Could you check a few things on this model? Use its own coordinates, in mm. Face numbers are marked on the shaded views. A direction names the side the tool comes from. Give positions to 0.01 mm unless a question says otherwise; leave off trailing zeros. Write each loop counter-clockwise with the first axis right and the second up, starting at its lowest first coordinate (ties: lowest second). Pieces come first, ordered by that corner, then holes. Notation, with made-up numbers: (-3.75, 39.5) -> (30.25, 39.5) arc R13 ccw to (30.25, 51.5) -> close; hole circle Ø4 at (17.25, -20.75). An arc over 180 degrees is marked (long way). One line per question, with ' | ' between items.
from build123d import *

# Parameters (mm, degrees)
ESQUISSE1_R             = 1.5
BOSS_EXTRU_1_DEPTH      = 4
ENL_V_MAT_EXTRU_1_REACH = 23.101


with BuildPart() as part:
    # Esquisse1 → Boss.-Extru.1 (new body)
    with BuildSketch(Plane.XY):
        with BuildLine():
            Line((0, 3), (17.5, 3))
            ThreePointArc((17.5, 3), (20.5, 0), (17.5, -3))
            Line((17.5, -3), (0, -3))
            ThreePointArc((0, -3), (-3, 0), (0, 3))
        make_face()
        Circle(ESQUISSE1_R, mode=Mode.SUBTRACT)
        with Locations((17.5, 0)):
            Circle(ESQUISSE1_R, mode=Mode.SUBTRACT)
    extrude(amount=BOSS_EXTRU_1_DEPTH)

    # Esquisse2 → Enlèv. mat.-Extru.1 (cut, up to next)
    with BuildSketch(Plane.XY.offset(4), mode=Mode.PRIVATE) as enl_v_mat_extru_1_sk1:
        with BuildLine():
            Line((4.5, 1), (13, 1))
            ThreePointArc((13, 1), (14, 0), (13, -1))
            Line((13, -1), (4.5, -1))
            ThreePointArc((4.5, -1), (3.5, 0), (4.5, 1))
        make_face()
    enl_v_mat_extru_1_tool1 = extrude(enl_v_mat_extru_1_sk1.sketch, amount=-ENL_V_MAT_EXTRU_1_REACH, mode=Mode.PRIVATE) & part.part
    add(enl_v_mat_extru_1_tool1.solids().sort_by_distance((8.75, 0, 4))[0], mode=Mode.SUBTRACT)


solid = part.part
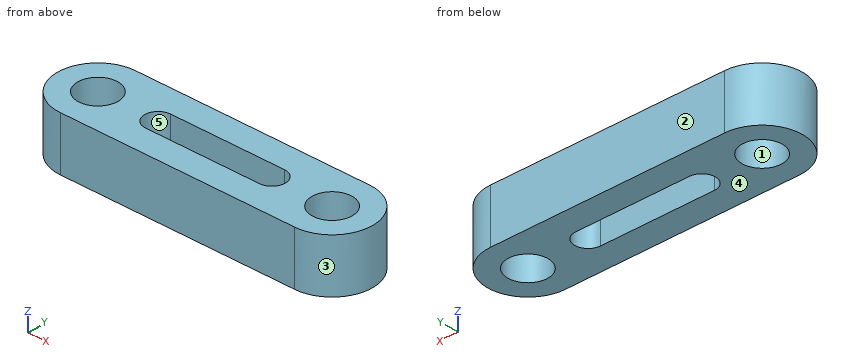
Q1. Imagine slicing it at B-B on x = 8.25. Please give me the cut outline in (y, z), and give its area (3 significant figures).
Answer below:
outline: (-3, 0) -> (-1, 0) -> (-1, 4) -> (-3, 4) -> close; (1, 0) -> (3, 0) -> (3, 4) -> (1, 4) -> close | area: 16.0 mm^2
Q2. Will this pin go through, and if not, where does the flat tip stop? pin 1 (1 mm diameter, centred on y = 2.5, z = 1.5, fed in from -X).
Answer below:
pin 1: stops at x = -2.24
Q3. Imagine slicing it at A-A on y = 0. Please give me the cut outline in (x, z), and give its area (3 significant figures).
Answer below:
outline: (-3, 0) -> (-1.5, 0) -> (-1.5, 4) -> (-3, 4) -> close; (1.5, 0) -> (3.5, 0) -> (3.5, 4) -> (1.5, 4) -> close; (14, 0) -> (16, 0) -> (16, 4) -> (14, 4) -> close; (19, 0) -> (20.5, 0) -> (20.5, 4) -> (19, 4) -> close | area: 28.0 mm^2
Q4. If we mould it in two halves opening along X, with no side actions, what happens to the marked faces 1, 2 and 3? For each: +X half, -X half, draft (parallel to the pull), parting line (faces both ways), or undercut.
Answer below:
face 1: undercut | face 2: draft | face 3: +X half
Q5. On a 3-axis mill with a long thin cutter (end or side, diameter ignored), from which of +Z, -Z, +X, -X, +Y, -Y can I reach the whole of each face in a straight line? I mean the marked faces 4 and 5. Say none if no direction works.
Answer below:
face 4: -Z, +X, -X, +Y, -Y | face 5: +Z, -Z
Q6. Imagine slicing it at D-D on y = 1.9. Please give me the cut outline in (x, z).
Answer below:
outline: (-2.32, 0) -> (19.82, 0) -> (19.82, 4) -> (-2.32, 4) -> close
Q7. Imagine slicing it at C-C on z = 0.45. Please give me the cut outline in (x, y), and give its area (3 significant figures).
Answer below:
outline: (0, -3) -> (17.5, -3) arc R3 ccw to (17.5, 3) -> (0, 3) arc R3 ccw to start; hole circle Ø3 at (0, 0); hole (4.5, -1) -> (13, -1) arc R1 ccw to (13, 1) -> (4.5, 1) arc R1 ccw to start; hole circle Ø3 at (17.5, 0) | area: 99.0 mm^2
Q8. If I drill on line 1 along Y through (x, z) = (5.75, 2.95); line 2 along X through (y, z) = (-0.7, 0.2); line 3 along Y through (x, z) = (17.5, 3.2), over which ranges is the centre line in solid material (lowest first)?
Answer below:
line 1: y = -3 to -1, 1 to 3 | line 2: x = -2.92 to -1.33, 1.33 to 3.79, 13.71 to 16.17, 18.83 to 20.42 | line 3: y = -3 to -1.5, 1.5 to 3
